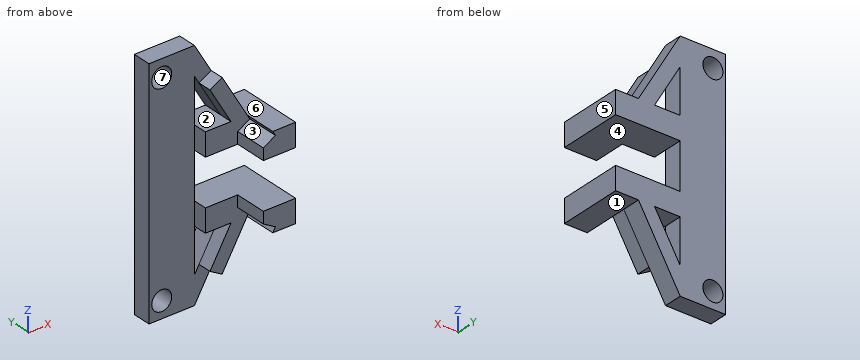
```python
from build123d import *

# Parameters (mm, degrees)
SKETCH1_R           = 1.375
BOSS_EXTRUDE1_DEPTH = 2.54
BOSS_EXTRUDE3_DEPTH = 1.905
BOSS_EXTRUDE4_DEPTH = 6.35


with BuildPart() as part:
    # Sketch1 → Boss-Extrude1 (new body)
    with BuildSketch(Plane(origin=(0, 0, 0), x_dir=(1, 0, 0), z_dir=(0, 1, 0))):
        Polygon((4.5, -2.375), (10.244923854, 7.5755), (13.39, 7.5755), (13.39, 10.7505), (4.5, 10.7505), (4.5, 17.1005), (13.39, 17.1005), (13.39, 20.2755), (10.244923854, 20.2755), (4.5, 30.226), (-1.75, 30.226), (-1.75, -2.375), align=None)
        with Locations(Location((0, 0, 0), (0, 0, 270))):
            Circle(SKETCH1_R, mode=Mode.SUBTRACT)
        Polygon((4.5, 7.5755), (8.028456448, 7.5755), (4.5, 1.46403416), align=None, mode=Mode.SUBTRACT)
        with Locations(Location((0, 27.94, 0), (0, 0, 270))):
            Circle(SKETCH1_R, mode=Mode.SUBTRACT)
        Polygon((4.5, 26.38696584), (8.028456448, 20.2755), (4.5, 20.2755), align=None, mode=Mode.SUBTRACT)
    extrude(amount=BOSS_EXTRUDE1_DEPTH)

    # Sketch1_3 → Boss-Extrude3 (add)
    with BuildSketch(Plane(origin=(0, 0, 0), x_dir=(1, 0, 0), z_dir=(0, 1, 0))):
        Polygon((13.39, 10.7505), (8.945, 10.7505), (8.945, 9.163), (10.607350554, 8.20324146), (10.244923854, 7.5755), (13.39, 7.5755), align=None)
        Polygon((8.945, 10.7505), (4.5, 10.7505), (4.5, 7.5755), (8.028456448, 7.5755), (8.945, 9.163), align=None)
        Polygon((8.028456448, 7.5755), (5.135, 2.563886423), (6.797350554, 1.604127883), (10.244923854, 7.5755), (8.945, 7.5755), align=None)
        Polygon((10.607350554, 8.20324146), (8.945, 9.163), (8.945, 7.5755), (10.244923854, 7.5755), align=None)
        Polygon((8.945, 9.163), (8.028456448, 7.5755), (8.945, 7.5755), align=None)
        Polygon((13.39, 20.2755), (10.244923854, 20.2755), (10.607350554, 19.64775854), (8.945, 18.688), (8.945, 17.1005), (13.39, 17.1005), align=None)
        Polygon((8.028456448, 20.2755), (4.5, 20.2755), (4.5, 17.1005), (8.945, 17.1005), (8.945, 18.688), align=None)
        Polygon((8.945, 18.688), (8.945, 20.2755), (8.028456448, 20.2755), align=None)
        Polygon((10.607350554, 19.64775854), (10.244923854, 20.2755), (8.945, 20.2755), (8.945, 18.688), align=None)
        Polygon((10.244923854, 20.2755), (6.797350554, 26.246872117), (5.135, 25.287113577), (8.028456448, 20.2755), (8.945, 20.2755), align=None)
    extrude(amount=-BOSS_EXTRUDE3_DEPTH)

    # Sketch1_4 → Boss-Extrude4 (add)
    with BuildSketch(Plane(origin=(0, 0, 0), x_dir=(1, 0, 0), z_dir=(0, 1, 0))):
        Polygon((13.39, 20.2755), (10.244923854, 20.2755), (10.607350554, 19.64775854), (8.945, 18.688), (8.945, 17.1005), (13.39, 17.1005), align=None)
        Polygon((13.39, 10.7505), (8.945, 10.7505), (8.945, 9.163), (10.607350554, 8.20324146), (10.244923854, 7.5755), (13.39, 7.5755), align=None)
    extrude(amount=-BOSS_EXTRUDE4_DEPTH)


solid = part.part
```
Check sheet for the modelled part. Datum: model origin and axes. Units: mm. Face numbers are marked on the shaded views. A direction names the side the tool comes from. Round coordinates to 2 decimals unless told otherwise and drop trailing zeros. Order: outer loops, then holes, each group sorted by start corner. A loop starts at its lowest first (then second) coordinate and runs counter-clockwise, first axis right, second up.
1) Section check C-C (z = -22.5). Record the boundary of the cut face in (x, y) (3 decimals), and give its area (3 significant figures).
2) Section check A-A (x = 0). Record the boundary of the cut face in (y, z) (3 decimals).
3) Section check D-D (x = 8.5). Record the boundary of the cut face in (y, z) (1 decimal).
4) Tool access check on the marked faces 1, 2, 3 and 4. Record the directions out of +Z, -Z, +X, -X, +Y, -Y that give a thin tool (end or side, any length) a straight path to the whole face; none if there is none.
5) Go/stop test with flat-tipped pins: pin 1 Ø2 at (y, z) = (1, -22.5) entering from +X; pin 2 Ø3 at (x, z) = (0, 0) entering from -Y; pin 3 Ø0.9 at (x, y) = (12.5, -3.5) entering from -Z. Record where each tip stops, or that it passes through.
6) Section check B-B (y = -3). Record the boundary of the cut face in (x, z) (1 decimal).
7) Scan lines: line 1 (Z direction, x = 12.75, y = 1); line 2 (X direction, y = 0.9, z = 0) (3 decimals); line 3 (X direction, y = 0.5, z = -25). Record each from-to range of solid material in increasing order.
8) Mould release check, pull along Z, two halves, no side actions. Record for the marked faces 5, 6 and 7: +Z half, -Z half, draft (parallel to the pull), parting line (faces both ways), or undercut.
Result:
1. outline: (-1.75, 0) - (4.5, 0) - (4.5, 2.54) - (-1.75, 2.54) - close; (6.744, -1.905) - (8.961, -1.905) - (8.961, 2.54) - (6.744, 2.54) - close
1. area: 25.7 mm2
2. outline: (0, -30.226) - (2.54, -30.226) - (2.54, -29.315) - (0, -29.315) - close; (0, -26.565) - (2.54, -26.565) - (2.54, -1.375) - (0, -1.375) - close; (0, 1.375) - (2.54, 1.375) - (2.54, 2.375) - (0, 2.375) - close
3. outline: (-1.9, -23.3) - (2.5, -23.3) - (2.5, -17.1) - (-1.9, -17.1) - close; (-1.9, -10.8) - (2.5, -10.8) - (2.5, -4.6) - (-1.9, -4.6) - close
4. face 1: -Z, +X, +Y, -Y
4. face 2: +Y, -Y
4. face 3: -X, -Y
4. face 4: +X, +Y, -Y
5. pin 1: stops at x = 9.54
5. pin 2: stops at y = 0
5. pin 3: stops at z = -20.28
6. outline: (8.9, -18.7) - (10.6, -19.6) - (10.2, -20.3) - (13.4, -20.3) - (13.4, -17.1) - (8.9, -17.1) - close; (8.9, -10.8) - (13.4, -10.8) - (13.4, -7.6) - (10.2, -7.6) - (10.6, -8.2) - (8.9, -9.2) - close
7. line 1: z = -20.28 to -17.1, -10.75 to -7.58
7. line 2: x = -1.75 to -1.375, 1.375 to 5.871
7. line 3: x = -1.75 to 4.5, 5.3 to 7.52
8. face 5: draft
8. face 6: +Z half
8. face 7: undercut
